Check sheet for the modelled part. Datum: model origin and axes. Units: mm. Face numbers are marked on the shaded views. Coordinates: 2 decimals unless noted, no trailing zeros. Write each loop counter-clockwise with the first axis right and the second up, starting at its lowest first coordinate (ties: lowest second). Pieces come first, ordered by that corner, then holes. Notation, with made-up numbers: (3.25, 32.5) - (25.25, 32.5) arc R27 ccw to (25.25, 57.5) - close; hole circle Ø7 at (60, 54). An arc over 180 degrees is marked (long way). Answer as CSV lines item,"result". Start each with the question number.
from build123d import *

# Parameters (mm, degrees)
BOSS_EXTRUDE1_DEPTH     = 0.7
SKETCH2_W               = 166.2
SKETCH2_H               = 100.6
BOSS_EXTRUDE2_DEPTH     = 5.26
SKETCH3_W               = 15
SKETCH3_H               = 8
BOSS_EXTRUDE3_DEPTH     = 2.5
CUT_EXTRUDE1_DEPTH      = 134.052151054
CUT_EXTRUDE1_DEPTH_BACK = 134.052151054
CUT_EXTRUDE2_REACH      = 113.566
SKETCH5_R               = 1.5


with BuildPart() as part:
    # Sketch1 → Boss-Extrude1 (new body)
    with BuildSketch(Plane.XY):
        with BuildLine():
            Line((-88.6, 55.38), (88.6, 55.38))
            ThreePointArc((88.6, 55.38), (94.172001436, 53.072001436), (96.48, 47.5))
            Line((96.48, 47.5), (96.48, -47.5))
            ThreePointArc((96.48, -47.5), (94.172001436, -53.072001436), (88.6, -55.38))
            Line((88.6, -55.38), (-88.6, -55.38))
            ThreePointArc((-88.6, -55.38), (-94.172001436, -53.072001436), (-96.48, -47.5))
            Line((-96.48, -47.5), (-96.48, 47.5))
            ThreePointArc((-96.48, 47.5), (-94.172001436, 53.072001436), (-88.6, 55.38))
        make_face()
    extrude(amount=BOSS_EXTRUDE1_DEPTH)

    # Sketch2 → Boss-Extrude2 (add)
    with BuildSketch(Plane.XY.offset(0.7)):
        with Locations((-1.49, -1.55)):
            Rectangle(SKETCH2_W, SKETCH2_H)
    extrude(amount=BOSS_EXTRUDE2_DEPTH)

    # Sketch3 → Boss-Extrude3 (add)
    with BuildSketch(Plane.XY.offset(5.96)):
        with Locations((-64.59, 33.8)):
            Rectangle(SKETCH3_W, SKETCH3_H)
        with Locations((-64.59, -31.85)):
            Rectangle(SKETCH3_W, SKETCH3_H)
        with Locations((61.61, 33.8)):
            Rectangle(SKETCH3_W, SKETCH3_H)
        with Locations((61.61, -31.85)):
            Rectangle(SKETCH3_W, SKETCH3_H)
    extrude(amount=BOSS_EXTRUDE3_DEPTH)

    # Sketch4 → Cut-Extrude1 (cut, two sides: drawn at the far end of the back side and taken through both)
    with BuildSketch(Plane.XZ.offset(35.85).offset(-CUT_EXTRUDE1_DEPTH_BACK)):
        Polygon((-72.09, 8.46), (-72.09, 5.96), (-69.09, 8.46), align=None)
        Polygon((-57.09, 5.96), (-57.09, 8.46), (-60.09, 8.46), align=None)
        Polygon((-60.452049935, 7.46), (-68.727950065, 7.46), (-70.527950065, 5.96), (-58.652049935, 5.96), align=None)
        Polygon((55.672049935, 5.96), (57.472049935, 7.46), (65.747950065, 7.46), (67.547950065, 5.96), align=None)
        Polygon((57.11, 8.46), (54.11, 5.96), (54.11, 8.46), align=None)
        Polygon((66.11, 8.46), (69.11, 8.46), (69.11, 5.96), align=None)
    extrude(amount=CUT_EXTRUDE1_DEPTH + CUT_EXTRUDE1_DEPTH_BACK, mode=Mode.SUBTRACT)

    # Sketch5 → Cut-Extrude2 (cut, up to next)
    with BuildSketch(Plane.XY.offset(8.46), mode=Mode.PRIVATE) as cut_extrude2_sk1:
        with Locations((-64.59, 33.8)):
            Circle(SKETCH5_R)
    cut_extrude2_tool1 = extrude(cut_extrude2_sk1.sketch, amount=-CUT_EXTRUDE2_REACH, mode=Mode.PRIVATE) & part.part
    # Sketch5 → Cut-Extrude2 (cut, up to next)
    with BuildSketch(Plane.XY.offset(8.46), mode=Mode.PRIVATE) as cut_extrude2_sk2:
        with Locations((-64.59, -31.85)):
            Circle(SKETCH5_R)
    cut_extrude2_tool2 = extrude(cut_extrude2_sk2.sketch, amount=-CUT_EXTRUDE2_REACH, mode=Mode.PRIVATE) & part.part
    # Sketch5 → Cut-Extrude2 (cut, up to next)
    with BuildSketch(Plane.XY.offset(8.46), mode=Mode.PRIVATE) as cut_extrude2_sk3:
        with Locations((61.61, -31.85)):
            Circle(SKETCH5_R)
    cut_extrude2_tool3 = extrude(cut_extrude2_sk3.sketch, amount=-CUT_EXTRUDE2_REACH, mode=Mode.PRIVATE) & part.part
    # Sketch5 → Cut-Extrude2 (cut, up to next)
    with BuildSketch(Plane.XY.offset(8.46), mode=Mode.PRIVATE) as cut_extrude2_sk4:
        with Locations((61.61, 33.8)):
            Circle(SKETCH5_R)
    cut_extrude2_tool4 = extrude(cut_extrude2_sk4.sketch, amount=-CUT_EXTRUDE2_REACH, mode=Mode.PRIVATE) & part.part
    add(cut_extrude2_tool1.solids().sort_by_distance((-64.59, 33.8, 8.46))[0], mode=Mode.SUBTRACT)
    add(cut_extrude2_tool2.solids().sort_by_distance((-64.59, -31.85, 8.46))[0], mode=Mode.SUBTRACT)
    add(cut_extrude2_tool3.solids().sort_by_distance((61.61, -31.85, 8.46))[0], mode=Mode.SUBTRACT)
    add(cut_extrude2_tool4.solids().sort_by_distance((61.61, 33.8, 8.46))[0], mode=Mode.SUBTRACT)


solid = part.part
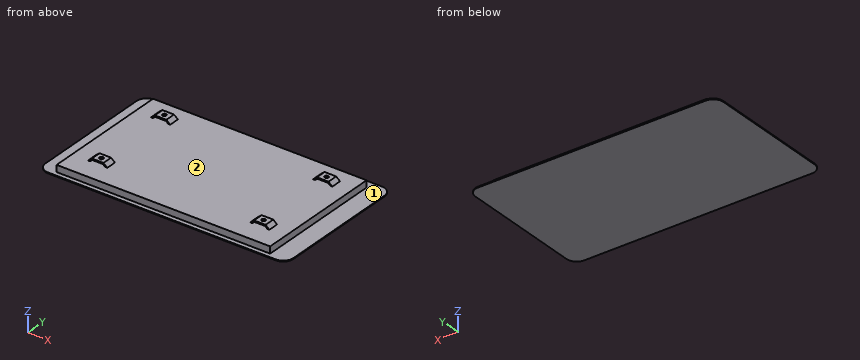
(1) Material ranges on probe 1 along Y at (x, z) = (-64.59, 7.75); probe 2 along X at (y, z) = (-13, 5.75); probe 3 along Z at (x, y) = (-57, 2.5), recorded low to high. Write a range as from..to.
(2) Go/stop test with flat-tipped pins: P1, Ø0.8, axis at x = 60.5, z = 6.5, coming from the -Y side; P2, Ø3, axis at x = -64, z = 7, coming from the +Y side; P3, Ø0.8, axis at x = 60, z = 8, coming from the +Y side; P4, Ø2, axis at x = -58, z = 3.5, coming from the -Y side. Record where each tip stops, or that it passes through.
(3) Cross-section at C-C on z = 4.5. Record the boundary of the cut face in (x, y), plus the area to 3 significant figures.
(4) Cross-section at A-A on x = 74. Record the boundary of the cut face in (y, z).
(5) Release check for a two-part mould opening along X. For the marked faces 1 and 2 record: pulls with the +X half, pulls with the -X half, needs draft (parallel to the pull), parting line crosses it, or undercut.
(6) Cross-section at B-B on y = -43.5. Record the boundary of the cut face in (x, z), plus the area to 3 significant figures.
Checked values:
1,probe 1,"-35.85..-33.35, -30.35..-27.85, 29.8..32.3, 35.3..37.8"
1,probe 2,"-84.59..81.61"
1,probe 3,"0..5.96"
2,P1,"through"
2,P2,"y = 48.75"
2,P3,"y = 37.8"
2,P4,"y = -51.85"
3,outline,"(-84.59, -51.85) - (81.61, -51.85) - (81.61, 48.75) - (-84.59, 48.75) - close"
3,area,"16,700 mm^2"
4,outline,"(-55.38, 0) - (55.38, 0) - (55.38, 0.7) - (48.75, 0.7) - (48.75, 5.96) - (-51.85, 5.96) - (-51.85, 0.7) - (-55.38, 0.7) - close"
5,face 1,"needs draft"
5,face 2,"undercut"
6,outline,"(-96.48, 0) - (96.48, 0) - (96.48, 0.7) - (81.61, 0.7) - (81.61, 5.96) - (-84.59, 5.96) - (-84.59, 0.7) - (-96.48, 0.7) - close"
6,area,"1,010 mm^2"
